Geometry: final body of the model. Coordinates: model frame, mm. Face numbers are marked on the shaded views. A direction names the side the tool comes from. Give positions to 0.01 mm unless a question says otherwise; leave off trailing zeros. Order: outer loops, then holes, each group sorted by start corner. A loop starts at its lowest first (then second) coordinate and runs counter-clockwise, first axis right, second up. Notation, with made-up numbers: (74, -35.5) - (82, -35.5) arc R25 cw to (82, -21.5) - close; hole circle Ø6 at (-18.5, 25). An arc over 180 degrees is marked (long way). Write item = value, one per line. Start each with the question number.
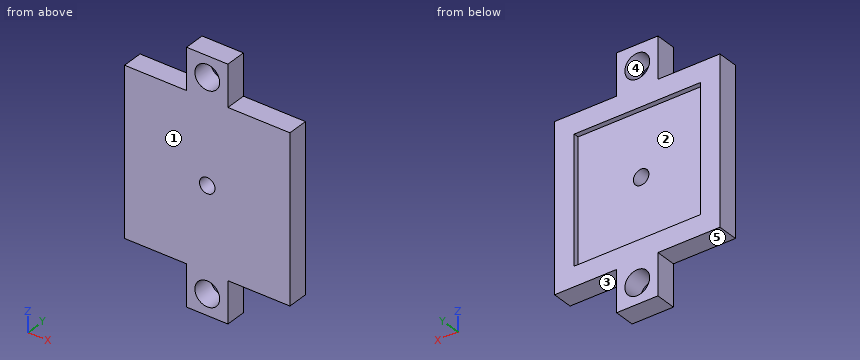
Autodesk Inventor part; units mm, degrees
ref_plane "YZ Plane" through (0, 0, 0) normal (1, 0, 0) x (0, 1, 0)
ref_plane "XZ Plane" through (0, 0, 0) normal (0, 1, 0) x (-1, 0, 0)
ref_plane "XY Plane" through (0, 0, 0) normal (0, 0, 1) x (1, 0, 0)
sketch "Sketch1" plane through (0, 0, 0) normal (0, 1, 0) x (-1, 0, 0)
  line L0 (0, 0) -> (-16, 0)
  line L1 (-16, 0) -> (-16, -16)
  line L2 (-16, -16) -> (0, -16)
  line L3 (0, -16) -> (0, 0)
  dimension "d0" = 16
  dimension "d1" = 16
extrude "Extrusion1" add sketch "Sketch1" along normal blind 1
sketch "Sketch5" plane through (0, 1, 0) normal (0, 1, 0) x (1, 0, 0)
  line L0 (16, 0) -> (16, 16)
  line L1 (0, 0) -> (16, 0)
  line L2 (16, 0) -> (16, 16)
  line L3 (16, 16) -> (0, 16)
  line L4 (0, 16) -> (0, 0)
  line L5 (0, 16) -> (0, 0)
  line L6 (0, 0) -> (1, 0)
  line L7 (1, 0) -> (1, 1)
  line L8 (1, 1) -> (0, 1)
  line L9 (0, 1) -> (0, 0)
  line L10 (16, 16) -> (0, 16)
  line L11 (16, 16) -> (15, 16)
  line L12 (15, 16) -> (15, 15)
  line L13 (15, 15) -> (16, 15)
  line L14 (16, 15) -> (16, 16)
  line L15 (15, 15) -> (1, 15)
  line L16 (1, 15) -> (1, 1)
  line L17 (1, 1) -> (15, 1)
  line L18 (15, 1) -> (15, 15)
  dimension "d20" = 1
  dimension "d21" = 1
  dimension "d22" = 1
  dimension "d23" = 1
extrude "Extrusion5" add sketch "Sketch5" along normal blind 1 contours L1 L7 L17 L18 L13 L0 | L13 L12 L3 L0 | L1 L4 L8 L7 | L15 L16 L8 L4 L3 L12
sketch "Sketch6" plane through (0, 1, 0) normal (0, 1, 0) x (1, 0, 0)
  line L0 (1, 1) -> (1, 15)
  line L1 (15, 15) -> (15, 1)
  line L2 (1, 15) -> (15, 15)
  line L3 (15, 1) -> (1, 1)
  circle A0 centre (8, 8) radius 0.75
  line L4 (1, 8) -> (7.25, 8)
  line L5 (8.75, 8) -> (15, 8)
  line L6 (8, 15) -> (8, 8.75)
  line L7 (8, 7.25) -> (8, 1)
  point P0 (0, 0)
  dimension "d26" = 1.5
extrude "Extrusion6" cut sketch "Sketch6" against normal blind 1 contours A0
sketch "Sketch9" plane through (0, 0, 0) normal (0, -1, 0) x (1, 0, 0)
  circle A0 centre (8, -8) radius 0.75
  line L0 (8, -8) -> (8, 0)
  line L1 (8, 0) -> (6, 0)
  line L2 (0, 0) -> (16, 0)
  line L3 (6, 0) -> (10, 0)
  line L4 (10, 0) -> (10, 4)
  line L5 (10, 4) -> (6, 4)
  line L6 (6, 4) -> (6, 0)
  line L7 (16, -16) -> (0, -16)
  line L8 (8, -16) -> (6, -16)
  line L9 (6, -16) -> (10, -16)
  line L10 (10, -16) -> (10, -20)
  line L11 (10, -20) -> (6, -20)
  line L12 (6, -20) -> (6, -16)
  circle A1 centre (8, 2) radius 1.2
  circle A2 centre (8, -18) radius 1.2
  dimension "d35" = 2
  dimension "d36" = 4
  dimension "d37" = 4
  dimension "d38" = 2
  dimension "d39" = 4
  dimension "d40" = 4
  dimension "d43" = 2.4
  dimension "d44" = 2.4
extrude "Extrusion9" add sketch "Sketch9" against normal blind 2 contours L1 L6 L5 L4 L2 | L10 L11 L12 L7
sketch "Sketch11" plane through (0, 1, 0) normal (0, 1, 0) x (1, 0, 0)
  line L0 (1, 1) -> (1, 15)
  line L1 (1, 1) -> (15, 1)
  line L2 (15, 1) -> (15, 15)
  line L3 (15, 15) -> (1, 15)
  line L4 (1, 15) -> (1, 1)
  line L5 (1, 1) -> (1.9, 1)
  line L6 (1.9, 1) -> (1.9, 1.9)
  line L7 (1.9, 1.9) -> (1, 1.9)
  line L8 (1, 1.9) -> (1, 1)
  line L9 (15, 1) -> (15, 15)
  line L10 (15, 15) -> (14.1, 15)
  line L11 (14.1, 15) -> (14.1, 14.1)
  line L12 (14.1, 14.1) -> (15, 14.1)
  line L13 (15, 14.1) -> (15, 15)
  line L14 (14.1, 14.1) -> (1.9, 14.1)
  line L15 (1.9, 14.1) -> (1.9, 1.9)
  line L16 (1.9, 1.9) -> (14.1, 1.9)
  line L17 (14.1, 1.9) -> (14.1, 14.1)
  point P0 (0, 0)
  dimension "d47" = 0.9
  dimension "d48" = 0.9
  dimension "d49" = 0.9
  dimension "d50" = 0.9
extrude "Extrusion10" add sketch "Sketch11" along normal blind 1 contours L0 L7 L6 L1 | L0 L3 L11 L14 L15 L7 | L6 L16 L17 L12 L2 L1 | L3 L2 L12 L11
sketch "Sketch12" plane through (0, 1, 0) normal (0, 1, 0) x (1, 0, 0)
  line L0 (1.9, 1.9) -> (1.9, 14.1)
  line L1 (14.1, 14.1) -> (14.1, 1.9)
  line L2 (1.9, 1.9) -> (14.1, 1.9)
  line L3 (14.1, 1.9) -> (14.1, 14.1)
  line L4 (14.1, 14.1) -> (1.9, 14.1)
  line L5 (1.9, 14.1) -> (1.9, 1.9)
  circle A0 centre (8, 8) radius 0.75
  circle A1 centre (8, 8) radius 0.75
  point P0 (0, 0)
  point P1 (14.1, 1.9)
  point P2 (1.9, 14.1)
extrude "Extrusion11" add sketch "Sketch12" along normal blind 0.5
properties part number "aruco_mount_v1"
Q1. Material intervals for line 1 along Z through (x, y) = (8, 0.75); line 2 along X through (y, z) = (0.55, -8); line 3 along X through (y, z) = (1.65, -3.5), sorted ascending. Write a range as from..to.
Q2. Section B-B, the plane x = 8. Return the cut outline in (y, z).
Q3. Pull-direction query (X, two-part tool) for the marked faces 4 and 5; classes: +X half, -X half, draft (parallel to the pull), parting line (faces both ways), or undercut.
Q4. Section D-D, the plane x = 9.75. Return the cut outline in (y, z).
Q5. Section A-A, the plane z = -8. Return the cut outline in (x, y), then the cut area to 4 significant figures.
Q6. Set-up query: the marked faces 1, 2 and 3. Return all of +Z, -Z, +X, -X, +Y, -Y with unobstructed straight access to the full face (end or side cutting, diameter ignored); none if empty.
Q7. Contact query for flat-ended pins moving along their axis: pin 1 (3 mm diameter, centred on x = 8, z = 2, fed in from -Y); pin 2 (1 mm diameter, centred on x = 14, y = 0.5, fed in from +Z); pin 3 (0.6 mm diameter, centred on y = 1.5, z = -17.5, fed in from +X); pin 4 (1 mm diameter, centred on x = 11.5, y = 0.5, fed in from -Z). Output: stop coordinate, or through.
Q8. Section C-C, the plane y = 0.5. Return the cut outline in (x, z), then the cut area to 3 significant figures.
The answers:
q1.line_1 = -20..-19.2, -16.8..-8.75, -7.25..0.8, 3.2..4
q1.line_2 = 0..7.25, 8.75..16
q1.line_3 = 0..1.9, 14.1..16
q2.outline = (0, -20) - (2, -20) - (2, -19.2) - (0, -19.2) - close; (0, -16.8) - (2, -16.8) - (2, -14.1) - (1.5, -14.1) - (1.5, -8.75) - (0, -8.75) - close; (0, -7.25) - (1.5, -7.25) - (1.5, -1.9) - (2, -1.9) - (2, 0.8) - (0, 0.8) - close; (0, 3.2) - (2, 3.2) - (2, 4) - (0, 4) - close
q3.face_4 = undercut
q3.face_5 = draft
q4.outline = (0, -20) - (2, -20) - (2, -14.1) - (1.5, -14.1) - (1.5, -1.9) - (2, -1.9) - (2, 4) - (0, 4) - close
q5.outline = (0, 0) - (7.25, 0) - (7.25, 1.5) - (1.9, 1.5) - (1.9, 2) - (0, 2) - close; (8.75, 0) - (16, 0) - (16, 2) - (14.1, 2) - (14.1, 1.5) - (8.75, 1.5) - close
q5.area = 23.65 mm²
q6.face_1 = +Z, -Z, +X, -X, -Y
q6.face_2 = +Y
q6.face_3 = -Z, +X, +Y, -Y
q7.pin_1 = 0
q7.pin_2 = 0
q7.pin_3 = 10
q7.pin_4 = -16
q8.outline = (0, -16) - (6, -16) - (6, -20) - (10, -20) - (10, -16) - (16, -16) - (16, 0) - (10, 0) - (10, 4) - (6, 4) - (6, 0) - (0, 0) - close; hole circle Ø2.4 at (8, -18); hole circle Ø2.4 at (8, 2); hole circle Ø1.5 at (8, -8)
q8.area = 277 mm²
